Part model, mm, in its own coordinate system. A direction names the side the tool comes from. Round coordinates to 2 decimals unless told otherwise and drop trailing zeros. Loops run counter-clockwise (first coordinate to the right, second up) from the corner with the lowest first, then second, coordinate; pieces in that order, holes last. Notation, with made-up numbers: (-16, 5.5) -> (-9, 5.5) arc R36 cw to (-9, 42.5) -> close; hole circle Ø9 at (53, 88). An arc over 180 degrees is marked (long way). Answer as a JSON object with one key per item and string values. Group by question number.
from build123d import *

# Parameters (mm, degrees)
SKETCH1_W           = 40
SKETCH1_H           = 50
BOSS_EXTRUDE1_DEPTH = 10
SKETCH2_W           = 60
SKETCH2_H           = 10
BOSS_EXTRUDE2_DEPTH = 20
FILLET1_R           = 10
SKETCH3_R           = 15
SKETCH3_R_2         = 10
BOSS_EXTRUDE3_DEPTH = 20
SKETCH4_R           = 6.5
CUT_EXTRUDE1_DEPTH  = 89.317608663


with BuildPart() as part:
    # Sketch1 → Boss-Extrude1 (new body)
    with BuildSketch(Plane.XY):
        Rectangle(SKETCH1_W, SKETCH1_H)
    extrude(amount=BOSS_EXTRUDE1_DEPTH)

    # Sketch2 → Boss-Extrude2 (add, symmetric)
    with BuildSketch(Plane(origin=(0, 0, 0), x_dir=(0, 0, -1), z_dir=(1, 0, 0))):
        with Locations((20, 30)):
            Rectangle(SKETCH2_W, SKETCH2_H)
        with Locations((20, -30)):
            Rectangle(SKETCH2_W, SKETCH2_H)
    extrude(amount=BOSS_EXTRUDE2_DEPTH, both=True)

    # Fillet1
    fillet1_edges = [part.edges().sort_by_distance(p)[0] for p in [
        (0, 35, 10),
        (-20, 30, -50),
        (20, 30, -50),
        (0, -35, 10),
        (-20, -30, -50),
        (20, -30, -50),
    ]]
    fillet(fillet1_edges, radius=FILLET1_R)

    # Sketch3 → Boss-Extrude3 (add)
    with BuildSketch(Plane.XY.offset(10)):
        with Locations(Location((0, 0, 0), (0, 0, 180))):
            Circle(SKETCH3_R)
        Circle(SKETCH3_R_2, mode=Mode.SUBTRACT)
    extrude(amount=BOSS_EXTRUDE3_DEPTH)

    # Sketch4 → Cut-Extrude1 (cut, through all)
    with BuildSketch(Plane(origin=(0, 35, 0), x_dir=(1, 0, 0), z_dir=(0, 1, 0))):
        with Locations(Location((0, 40, 0), (0, 0, 270))):
            Circle(SKETCH4_R)
    extrude(amount=-CUT_EXTRUDE1_DEPTH, mode=Mode.SUBTRACT)


solid = part.part
Item 1: Drop flat-ended pins along their axis: pin 1 Ø6 at (x, y) = (0, 1.5) entering from +Z; pin 2 Ø11.5 at (x, z) = (0, -40) entering from +Y; pin 3 Ø6 at (x, y) = (15, 23) entering from -Z. Give the stop position or say it passes through.
Item 2: Band-saw the part on C-C, the plane y = 0. List the corners of the cut face in (x, z), plus the area to 3 significant figures.
Item 3: Band-saw the part on A-A, the plane x = 0. List the corners of the cut face in (y, z), plus the area to 3 significant figures.
Item 4: Two-plate mould, pull along X, no slides. Class faces 1 (the face through (-0.28, 31.99, 7.15)), 2 (the face through (0, 0, 10)), 3 (the face through (0.286, 30.07, -46.494)), 4 (the face through (-16.99, 30.07, -47.15)): pulls with the +X half, pulls with the -X half, needs draft (parallel to the pull), parting line crosses it, or undercut.
Item 5: Drill centre lines: line 1 (Y direction, x = -3, z = -20); line 2 (X direction, y = 28, z = -40); line 3 (Y direction, x = 0, z = 15). Where is each one in solid material? Low to high.
Item 6: Band-saw the part on B-B, the plane z = -6. List the corners of the cut face in (x, y), plus the area to 3 significant figures.
Item 7: Band-saw the part on D-D, the plane y = 28.5. List the corners of the cut face in (x, z), plus the area to 3 significant figures.
Item 8: Which spindle directions (+Z, -Z, +X, -X, +Y, -Y) get a long thin tool onto all of the face, cutting with end or side? Do faces 5 (the face through (0, -25, -25)), 6 (the face through (-2.17, -9.76, 19.86)), 7 (the face through (0, -35, -25)). Say none if no direction does.
Entries:
{
 "1": {"pin 1": "z = 10", "pin 2": "through", "pin 3": "z = -49.61"},
 "2": {"outline": "(-20, 0) -> (20, 0) -> (20, 10) -> (15, 10) -> (15, 30) -> (10, 30) -> (10, 10) -> (-10, 10) -> (-10, 30) -> (-15, 30) -> (-15, 10) -> (-20, 10) -> close", "area": "600 mm²"},
 "3": {"outline": "(-35, -50) -> (-25, -50) -> (-25, -46.5) -> (-35, -46.5) -> close; (-35, -33.5) -> (-25, -33.5) -> (-25, 0) -> (25, 0) -> (25, -33.5) -> (35, -33.5) -> (35, 0) arc R10 ccw to (25, 10) -> (15, 10) -> (15, 30) -> (10, 30) -> (10, 10) -> (-10, 10) -> (-10, 30) -> (-15, 30) -> (-15, 10) -> (-25, 10) arc R10 ccw to (-35, 0) -> close; (25, -50) -> (35, -50) -> (35, -46.5) -> (25, -46.5) -> close", "area": "1,600 mm²"},
 "4": {"face 1": "needs draft", "face 2": "undercut", "face 3": "undercut", "face 4": "pulls with the -X half"},
 "5": {"line 1": "-35 to -25, 25 to 35", "line 2": "-20 to -6.5, 6.5 to 20", "line 3": "-15 to -10, 10 to 15"},
 "6": {"outline": "(-20, -35) -> (20, -35) -> (20, -25) -> (-20, -25) -> close; (-20, 25) -> (20, 25) -> (20, 35) -> (-20, 35) -> close", "area": "800 mm²"},
 "7": {"outline": "(-20, -40) arc R10 ccw to (-10, -50) -> (10, -50) arc R10 ccw to (20, -40) -> (20, 9.37) -> (-20, 9.37) -> close; hole circle Ø13 at (0, -40)", "area": "2,200 mm²"},
 "8": {"face 5": "-Z, +X, -X", "face 6": "+Z", "face 7": "+Z, -Z, +X, -X, -Y"}
}
